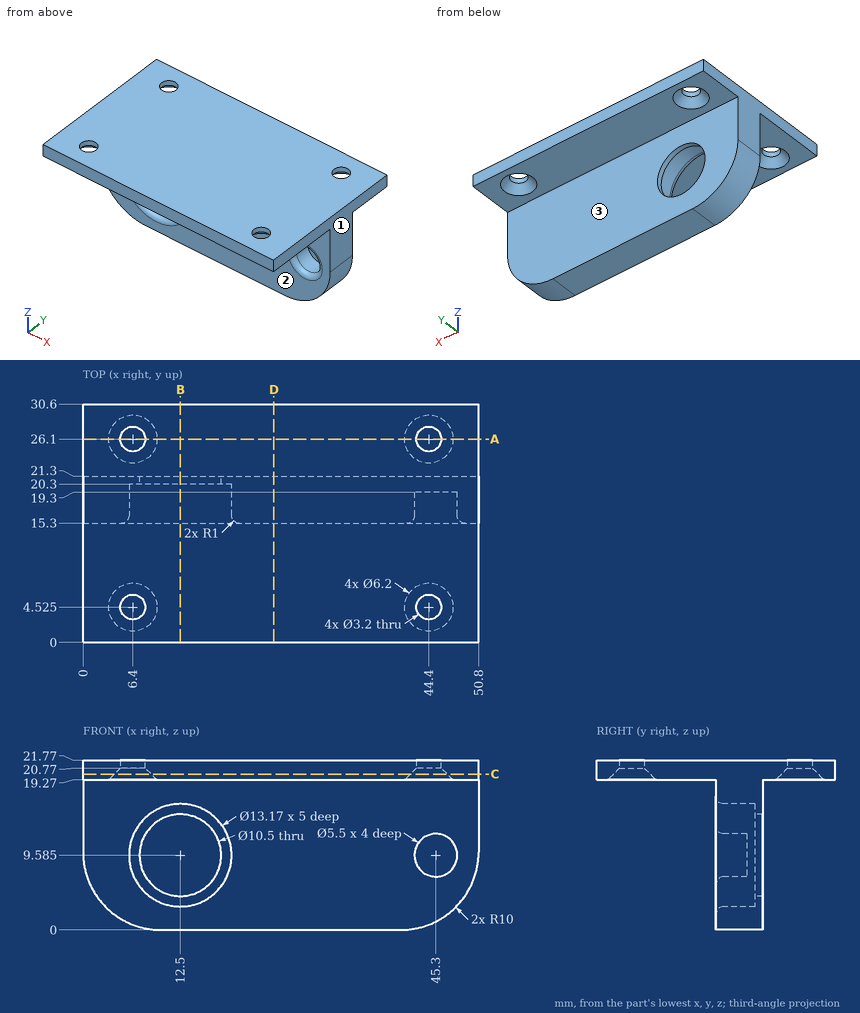
Could you check a few things on this drawing? It's one solid part, dimensions in mm from its lowest x, y, z. A direction names the side the tool comes from. Give positions to 0.01 mm unless a question says otherwise; leave off trailing zeros. Write each loop counter-clockwise with the first axis right and the second up, starting at its lowest first coordinate (ties: lowest second). Pieces come first, ordered by that corner, then holes. Notation, with made-up numbers: (68.25, 19) -> (88.25, 19) arc R19 cw to (88.25, 32) -> close; hole circle Ø7 at (26, -5). An arc over 180 degrees is marked (long way). Answer as a JSON object with one key per item and string values.
Q1. Suppose I cut it at D-D on x = 24.5. Write out the boundary of the cut face in (y, z), then the cut area to 3 significant figures.
Taken from the geometry:
{"outline": "(0, 19.27) -> (15.3, 19.27) -> (15.3, 0) -> (21.3, 0) -> (21.3, 19.27) -> (30.6, 19.27) -> (30.6, 21.77) -> (0, 21.77) -> close", "area": "192 mm²"}
Q2. Suppose I cut it at B-B on x = 12.5. Write out the boundary of the cut face in (y, z) (3 decimals).
Taken from the geometry:
{"outline": "(0, 19.27) -> (15.3, 19.27) -> (15.3, 17.17) arc R1 ccw to (16.3, 16.17) -> (20.3, 16.17) -> (20.3, 14.835) -> (21.3, 14.835) -> (21.3, 19.27) -> (30.6, 19.27) -> (30.6, 21.77) -> (0, 21.77) -> close; (15.3, 0) -> (21.3, 0) -> (21.3, 4.335) -> (20.3, 4.335) -> (20.3, 3) -> (16.3, 3) arc R1 ccw to (15.3, 2) -> close"}
Q3. Please list where these lines run through material, in increasing order: L1, parallel to Y at x = 6.4, z = 21.6 (3 decimals); L2, parallel to X at y = 26.1, z = 21.35; L3, parallel to Z at x = 37, y = 23.5.
Taken from the geometry:
{"L1": "y = 0 to 2.925, 6.125 to 24.5, 27.7 to 30.6", "L2": "x = 0 to 4.8, 8 to 42.8, 46 to 50.8", "L3": "z = 19.27 to 21.77"}
Q4. Suppose I cut it at C-C on z = 20. Write out the boundary of the cut face in (x, y) (3 decimals), then the cut area to 3 significant figures.
Taken from the geometry:
{"outline": "(0, 0) -> (50.8, 0) -> (50.8, 30.6) -> (0, 30.6) -> close; hole circle Ø4.74 at (6.4, 4.525); hole circle Ø4.74 at (6.4, 26.1); hole circle Ø4.74 at (44.4, 4.525); hole circle Ø4.74 at (44.4, 26.1)", "area": "1,480 mm²"}
Q5. Suppose I cut it at A-A on y = 26.1. Write out the boundary of the cut face in (x, z).
Taken from the geometry:
{"outline": "(0, 19.27) -> (3.3, 19.27) -> (4.8, 20.77) -> (4.8, 21.77) -> (0, 21.77) -> close; (8, 20.77) -> (9.5, 19.27) -> (41.3, 19.27) -> (42.8, 20.77) -> (42.8, 21.77) -> (8, 21.77) -> close; (46, 20.77) -> (47.5, 19.27) -> (50.8, 19.27) -> (50.8, 21.77) -> (46, 21.77) -> close"}
Q6. Will these pins go through, and if not, where does the flat tip stop? pin 1 Ø8 at (y, z) = (6.5, 17) entering from +X; pin 2 Ø3 at (x, y) = (6.4, 4.525) entering from -Z; pin 3 Ø4 at (x, y) = (44.4, 4.525) entering from -Z; pin 4 Ø3.5 at (x, y) = (44.4, 26.1) entering from -Z.
Taken from the geometry:
{"pin 1": "stops at x = 50.8", "pin 2": "passes through", "pin 3": "stops at z = 20.37", "pin 4": "stops at z = 20.62"}
Q7. Which directions (+Z, -Z, +X, -X, +Y, -Y) give clear straight access to the entire face, cutting with the end or side of a thin tool? Please do the marked faces 1, 2 and 3.
Taken from the geometry:
{"face 1": "+Z, -Z, +X, +Y, -Y", "face 2": "-Z, +X, -X, -Y", "face 3": "-Z, +X, -X, +Y"}
